```python
from build123d import *

# Parameters (mm, degrees)
SKETCH1_W           = 60
SKETCH1_H           = 40
BOSS_EXTRUDE1_DEPTH = 2
SKETCH4_W           = 10
SKETCH4_H           = 3
BOSS_EXTRUDE2_DEPTH = 8
SKETCH6_W           = 10
SKETCH6_H           = 8
BOSS_EXTRUDE5_DEPTH = 8
SKETCH8_R           = 2
CUT_EXTRUDE2_DEPTH  = 8
SKETCH9_W           = 20
SKETCH9_H           = 4
BOSS_EXTRUDE6_DEPTH = 4
SKETCH10_R          = 6.5
SKETCH10_R_2        = 2
BOSS_EXTRUDE7_DEPTH = 20
FILLET1_R           = 1
FILLET2_R           = 1
FILLET3_R           = 1


with BuildPart() as part:
    # Sketch1 → Boss-Extrude1 (new body)
    with BuildSketch(Plane(origin=(0, 0, 0), x_dir=(1, 0, 0), z_dir=(0, 1, 0))):
        Rectangle(SKETCH1_W, SKETCH1_H)
    extrude(amount=BOSS_EXTRUDE1_DEPTH)

    # Sketch3 → Loft1 section 0
    with BuildSketch(Plane(origin=(0, 22, 0), x_dir=(1, 0, 0), z_dir=(0, 1, 0))):
        with BuildLine():
            Line((-20.040616465, 5.303560218), (-10.040616465, 5.303560218))
            Line((-10.040616465, 5.303560218), (-10.040616465, 8.303560218))
            Line((-10.040616465, 8.303560218), (-20.040616465, 8.303560218))
            Line((-20.040616465, 8.303560218), (-20.040616465, 5.303560218))
        make_face()
    # Sketch2 → Loft1 section 1
    with BuildSketch(Plane(origin=(0, 2, 0), x_dir=(1, 0, 0), z_dir=(0, 1, 0))):
        with BuildLine():
            Line((-21.540616465, 5.303560218), (-8.540616465, 5.303560218))
            Line((-8.540616465, 5.303560218), (-8.540616465, 8.303560218))
            Line((-8.540616465, 8.303560218), (-21.540616465, 8.303560218))
            Line((-21.540616465, 8.303560218), (-21.540616465, 5.303560218))
        make_face()
    loft()

    # Sketch4 → Boss-Extrude2 (add)
    with BuildSketch(Plane(origin=(0, 22, 0), x_dir=(1, 0, 0), z_dir=(0, 1, 0))):
        with Locations((-15.040616465, 6.803560218)):
            Rectangle(SKETCH4_W, SKETCH4_H)
    extrude(amount=BOSS_EXTRUDE2_DEPTH)

    # Sketch6 → Boss-Extrude5 (add)
    with BuildSketch(Plane.XY.offset(-5.303560218)):
        with Locations((-15.040616465, 26)):
            Rectangle(SKETCH6_W, SKETCH6_H)
    extrude(amount=BOSS_EXTRUDE5_DEPTH)

    # Sketch8 → Cut-Extrude2 (cut)
    with BuildSketch(Plane(origin=(0, 30, 0), x_dir=(1, 0, 0), z_dir=(0, 1, 0))):
        with Locations(Location((-15.040616465, 1.048838028, 0), (0, 0, 270))):
            Circle(SKETCH8_R)
    extrude(amount=-CUT_EXTRUDE2_DEPTH, mode=Mode.SUBTRACT)

    # Sketch9 → Boss-Extrude6 (add)
    with BuildSketch(Plane(origin=(0, 2, 0), x_dir=(1, 0, 0), z_dir=(0, 1, 0))):
        with Locations((17.019567568, -8.907492708)):
            Rectangle(SKETCH9_W, SKETCH9_H)
    extrude(amount=BOSS_EXTRUDE6_DEPTH)

    # Sketch10 → Boss-Extrude7 (add)
    with BuildSketch(Plane(origin=(27.019567568, 0, 0), x_dir=(0, 0, -1), z_dir=(1, 0, 0))):
        with Locations((-8.907492708, 11.238036321)):
            Circle(SKETCH10_R)
        with Locations((-8.907492708, 11.238036321)):
            Circle(SKETCH10_R_2, mode=Mode.SUBTRACT)
    extrude(amount=-BOSS_EXTRUDE7_DEPTH)

    # Fillet1
    fillet1_edges = [part.edges().sort_by_distance(p)[0] for p in [
        (-21.540616465, 2, -6.803560218),
        (-15.040616465, 2, -5.303560218),
        (-15.040616465, 2, -8.303560218),
        (-8.540616465, 2, -6.803560218),
    ]]
    fillet(fillet1_edges, radius=FILLET1_R)

    # Fillet2
    fillet2_edges = [part.edges().sort_by_distance(p)[0] for p in [
        (-15.040616465, 22, -5.303560218),
    ]]
    fillet(fillet2_edges, radius=FILLET2_R)

    # Fillet3
    fillet3_edges = [part.edges().sort_by_distance(p)[0] for p in [
        (17.019567568, 2, 10.907492708),
        (27.019567568, 2, 8.907492708),
        (7.019567568, 2, 8.907492708),
        (17.019567568, 2, 6.907492708),
        (17.019567568, 5.053377883, 6.907492708),
        (17.019567568, 5.053377883, 10.907492708),
    ]]
    fillet(fillet3_edges, radius=FILLET3_R)


solid = part.part
```
Verification items for the finished model (mm, model axes). A direction names the side the tool comes from. Give positions to 0.01 mm unless a question says otherwise; leave off trailing zeros. Write each loop counter-clockwise with the first axis right and the second up, starting at its lowest first coordinate (ties: lowest second). Pieces come first, ordered by that corner, then holes. Notation, with made-up numbers: M -20.5,-23.5 L 3.5,-23.5 A26 ccw 3.5,8.5 Z; hole C -25,59.5 d1. An arc over 180 degrees is marked long. One line per question, with ' | ' between items.
1) Mould release check, pull along Z, two halves, no side actions. Record for faces 5 (the cylindrical face through (17.16, 17.733, 8.659)), 6 (the flat face through (17, 4, 6.907)), 7 (the cylindrical face through (17.16, 9.286, 9.341)): released by +Z, released by -Z, zero draft, split by the parting line, or undercut.
Result:
face 5: split by the parting line | face 6: released by -Z | face 7: undercut
2) Thickness scan on line 1 along Y through (x, z) = (-8, -13.5); line 2 along Z through (x, y) = (-15.5, 11.5); line 3 along X through (y, z) = (8.5, 7). Record the ranges inside material, lowest first. Write a range as [from, to].
Result:
line 1: y = [0, 2] | line 2: z = [-8.3, -5.3] | line 3: x = [7.02, 27.02]
3) Section check D-D on z = 8. Enter the section's corners in (x, y).
Result:
outline: M -30,0 L 30,0 L 30,2 L 28.02,2 A1 cw 27.02,3 L 27.02,9.46 L 7.02,9.46 L 7.02,3 A1 cw 6.02,2 L -30,2 Z; M 7.02,13.02 L 27.02,13.02 L 27.02,17.67 L 7.02,17.67 Z
4) Set-up check for faces 1 (the flat face through (-15, 16, -8.304)), 2 (the flat face through (-14, 22, 1)), 3 (the flat face through (7.02, 9, 9)), 4 (the flat face through (-10.041, 26, -3)): record each of +Z, -Z, +X, -X, +Y, -Y from which the full face is reachable in a straight line by a thin tool's end or side.
Result:
face 1: -Z, +X, -X, +Y | face 2: +Z, +X, -X | face 3: +Z, -Z, -X, +Y | face 4: +Z, -Z, +X, +Y
5) Section check A-A on z = -7. Enter the section's corners in (x, y).
Result:
outline: M -30,0 L 30,0 L 30,2 L -7.61,2 A1 cw -8.61,2.93 L -10.04,22 L -10.04,30 L -20.04,30 L -20.04,22 L -21.47,2.93 A1 cw -22.47,2 L -30,2 Z
6) Section check C-C on x = 20. Enter the section's corners in (y, z), plus the area to 3 significant figures.
Result:
outline: M 0,-20 L 2,-20 L 2,5.91 A1 cw 3,6.91 L 4.36,6.91 A1 cw 5.28,6.31 A6.5 ccw long 5.28,11.51 A1 cw 4.36,10.91 L 3,10.91 A1 cw 2,11.91 L 2,20 L 0,20 Z; hole C 11.24,8.91 d4 | area: 212 mm2
7) Section check B-B on z = -2. Enter the section's corners in (x, y).
Result:
outline: M -30,0 L 30,0 L 30,2 L -30,2 Z; M -20.04,22 L -16.8,22 L -16.8,30 L -20.04,30 Z; M -13.28,22 L -10.04,22 L -10.04,30 L -13.28,30 Z
8) Gauge pin test, flat ends, axial feed: pin 1 Ø1.1 at (x, y) = (18.5, 4) entering from -Z; pin 2 Ø2.5 at (y, z) = (25, -5) entering from -X; pin 3 Ø5 at (y, z) = (10.5, 15) entering from -X; pin 4 Ø1.5 at (y, z) = (9.5, -3.5) entering from -X. Record the tip position at first contact, or that the pin passes through.
Result:
pin 1: stops at z = 6.89 | pin 2: stops at x = -20.04 | pin 3: stops at x = 7.02 | pin 4: passes through
